For this review, use the dimensioned drawing (mm, ordinates from the lowest corner) and the shaded views. A direction names the side the tool comes from. Round coordinates to 2 decimals unless told otherwise and drop trailing zeros. Loops run counter-clockwise (first coordinate to the right, second up) from the corner with the lowest first, then second, coordinate; pieces in that order, holes last. Notation, with made-up numbers: M 9,-19 L 66,-19 A26 ccw 66,6 Z; hole C -40,-38.5 d6. An arc over 180 degrees is marked long. Answer as a JSON object with one key per item and string values. Group by question number.
Item 1: Tool access review of the marked faces 4, 5 and 6: name each direction out of +Z, -Z, +X, -X, +Y, -Y from which nothing blocks a thin tool from reaching the whole face with its end or side.
Item 2: The part is to be moulded in two halves that separate along X. For the marked faces 1, 2 and 3, say which applies: +X half, -X half, draft (parallel to the pull), parting line (faces both ways), or undercut.
Item 3: Consider section C-C (x = 8.25). Give the boundary of the cut face in (y, z), and give its area (3 significant figures).
Item 4: Insertion check: P1, Ø6, axis at x = 18.5, z = 2, coming from the -Y side; P2, Ø6, axis at x = 21.5, z = 12.5, coming from the -Y side. Each pin has a flat end and moves straight along its axis. Give the tip position at first contact, or say it passes through.
Item 5: To check wall thickness, follow line 1 (X direction, y = 6.5, z = 8); line 2 (Y direction, x = 24.75, z = 5); line 3 (Y direction, x = 15.5, z = 12.25). State the ranges of each line that lie inside material, in increasing order.
Item 6: Consider section A-A (y = 13.5). Give the boundary of the cut face in (x, z), and give its area (3 significant figures).
Item 7: Consider section B-B (z = 13.5). Give the boundary of the cut face in (x, y).
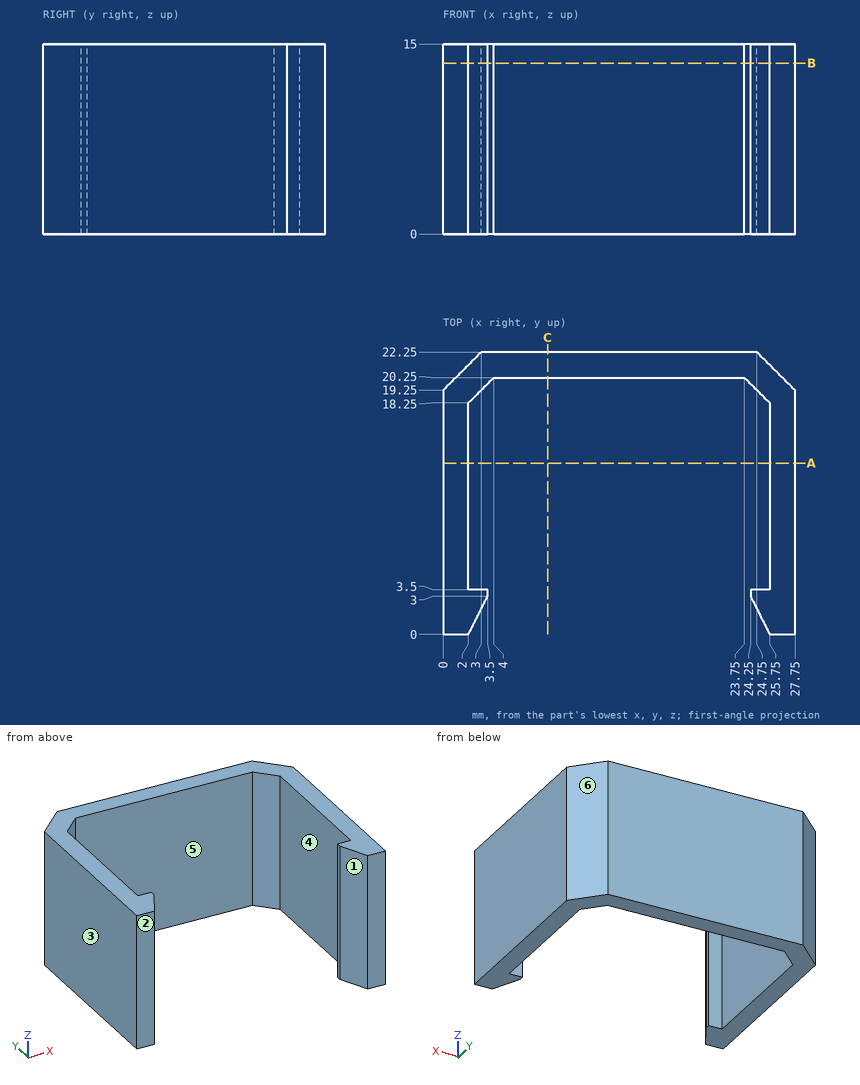
Geometry results:
{
 "1": {"face 4": "+Z, -Z", "face 5": "+Z, -Z, -Y", "face 6": "+Z, -Z, +X, +Y"},
 "2": {"face 1": "undercut", "face 2": "draft", "face 3": "-X half"},
 "3": {"outline": "M 20.25,0 L 22.25,0 L 22.25,15 L 20.25,15 Z", "area": "30.0 mm^2"},
 "4": {"P1": "stops at y = 20.25", "P2": "stops at y = 2.5"},
 "5": {"line 1": "x = 0 to 2, 25.75 to 27.75", "line 2": "y = 2 to 3.5, 19.25 to 22.25", "line 3": "y = 20.25 to 22.25"},
 "6": {"outline": "M 0,0 L 2,0 L 2,15 L 0,15 Z; M 25.75,0 L 27.75,0 L 27.75,15 L 25.75,15 Z", "area": "60.0 mm^2"},
 "7": {"outline": "M 0,0 L 2,0 L 3.5,3 L 3.5,3.5 L 2,3.5 L 2,18.25 L 4,20.25 L 23.75,20.25 L 25.75,18.25 L 25.75,3.5 L 24.25,3.5 L 24.25,3 L 25.75,0 L 27.75,0 L 27.75,19.25 L 24.75,22.25 L 3,22.25 L 0,19.25 Z"}
}
